Model file for the job. Use its own axes, mm. A direction names the side the tool comes from. Give positions to 0.01 mm unless a question says otherwise; leave off trailing zeros. Loops run counter-clockwise (first coordinate to the right, second up) from the corner with the lowest first, then second, coordinate; pieces in that order, holes last. Notation, with made-up numbers: (-12, 40) -> (35, 40) arc R23 ccw to (35, 60) -> close; hole circle Ø5 at (-21.75, 20.25). An arc over 180 degrees is marked (long way). Use CSV: the item, a comma, the result in double quotes. Start each with the question number.
(1) Pull direction X, two halves, no side cores. Call faces 5 (the flat face through (5, -37, -3)), 6 (the flat face through (0, -20, -22)), 7 (the flat face through (3, -37, 27.5)), 8 (the flat face through (-5, -37, -2)): pulls with the +X half, pulls with the -X half, needs draft (parallel to the pull), parting line crosses it, or undercut.
(2) 3-axis set-ups, long thin cutter, end or side, ignore diameter. For faces 1 (the cylindrical face through (-0.65, -65.14, -25.43)), 2 (the flat face through (0, -20, 23)), 3 (the cylindrical face through (-2.934, -35.548, -27.57)), 4 (the cylindrical face through (0.07, -48.974, -6.148)): which of +Z, -Z, +X, -X, +Y, -Y reach the whole face in a straight line?
(3) Flat gauge pins, fed straight in: pin 1 (2 mm diameter, centred on x = 2.5, y = -61, fed in from +Z); pin 2 (5.5 mm diameter, centred on x = 0, z = -22.5, fed in from +Y); pin 3 (3 mm diameter, centred on x = 1, z = -23, fed in from -Y). Where does each tip first touch, or does it go through?
(4) Cut at B-B on y = -18.5. Write the cut outline in (x, z).
(5) Drill centre lines: probe 1 along Y at (x, z) = (-2.5, -26.75); probe 2 along Z at (x, y) = (0.5, -15); probe 3 along Z at (x, y) = (2, -28). Where is each one in solid material? Low to high.
(6) Cut at A-A on z = -27.5. Write the cut outline in (x, y), then the cut area to 3 significant figures.
(7) Cut at D-D on y = -47.5. Write the cut outline in (x, z).
(8) Cut at C-C on z = -7.5. Write the cut outline in (x, y).
from build123d import *

# Parameters (mm, degrees)
F1_DEPTH  = 75
F3_R      = 2
F4_DEPTH  = 25
F6_R      = 3
F7_DEPTH  = 20
F8_R      = 3
F9_DEPTH  = 20
F10_R     = 3
F11_DEPTH = 20
F12_R     = 3
F13_DEPTH = 20
F2_R      = 2
F14_DEPTH = 10
F15_DEPTH = 25


with BuildPart() as f1:
    # F0 (on Front) → F1 (new body)
    with BuildSketch(Plane.XZ):
        Polygon((-5, 27.5), (-5, -32.5), (5, -32.5), (5, 27.5), (0, 27.5), (0, 32.5), align=None)
    extrude(amount=F1_DEPTH)

    # F3 (on face) → F4 (cut)
    with BuildSketch(Plane.YZ.offset(5)):
        with Locations((-47.5, -27.5)):
            Circle(F3_R)
        with Locations((-47.5, -7.5)):
            Circle(F3_R)
        with Locations((-27.5, -7.5)):
            Circle(F3_R)
        with Locations((-27.5, -27.5)):
            Circle(F3_R)
    extrude(amount=-F4_DEPTH, mode=Mode.SUBTRACT)

    # F6 (on face) → F7 (cut)
    with BuildSketch(Plane(origin=(0, 0, 0), x_dir=(-1, 0, 0), z_dir=(0, 1, 0))):
        with Locations((0, -22.5)):
            Circle(F6_R)
    extrude(amount=-F7_DEPTH, mode=Mode.SUBTRACT)

    # F8 (on face) → F9 (cut)
    with BuildSketch(Plane.XZ.offset(75)):
        with Locations((0, 22.5)):
            Circle(F8_R)
    extrude(amount=-F9_DEPTH, mode=Mode.SUBTRACT)

    # F10 (on face) → F11 (cut)
    with BuildSketch(Plane.XZ.offset(75)):
        with Locations((0, -22.5)):
            Circle(F10_R)
    extrude(amount=-F11_DEPTH, mode=Mode.SUBTRACT)

    # F12 (on face) → F13 (cut)
    with BuildSketch(Plane(origin=(0, 0, 0), x_dir=(-1, 0, 0), z_dir=(0, 1, 0))):
        with Locations((0, 22.5)):
            Circle(F12_R)
    extrude(amount=-F13_DEPTH, mode=Mode.SUBTRACT)

    # F2 (on face) → F14 (cut)
    with BuildSketch(Plane(origin=(0, 0, -32.5), x_dir=(1, 0, 0), z_dir=(0, 0, -1))):
        with Locations((-2.5, 37.5)):
            Circle(F2_R)
    extrude(amount=-F14_DEPTH, mode=Mode.SUBTRACT)

    # F3 (on face) → F15 (cut)
    with BuildSketch(Plane.YZ.offset(5)):
        with Locations((-47.5, -27.5)):
            Circle(F3_R)
        with Locations((-47.5, -7.5)):
            Circle(F3_R)
        with Locations((-27.5, -7.5)):
            Circle(F3_R)
        with Locations((-27.5, -27.5)):
            Circle(F3_R)
    extrude(amount=-F15_DEPTH, mode=Mode.SUBTRACT)


solid = f1.part
Check result:
1,face 5,"pulls with the +X half"
1,face 6,"undercut"
1,face 7,"needs draft"
1,face 8,"pulls with the -X half"
2,face 1,"-Y"
2,face 2,"+Y"
2,face 3,"-Z"
2,face 4,"+X, -X"
3,pin 1,"z = 27.5"
3,pin 2,"y = -20"
3,pin 3,"y = -55"
4,outline,"(-5, -32.5) -> (5, -32.5) -> (5, 27.5) -> (0, 27.5) -> (0, 32.5) -> (-5, 27.5) -> close; hole circle Ø6 at (0, -22.5); hole circle Ø6 at (0, 22.5)"
5,probe 1,"-75 to -49.35, -45.65 to -39.5, -35.5 to -29.35, -25.65 to 0"
5,probe 2,"-32.5 to -25.46, -19.54 to 19.54, 25.46 to 27.5"
5,probe 3,"-32.5 to -29.44, -25.56 to -9.44, -5.56 to 27.5"
6,outline,"(-5, -75) -> (5, -75) -> (5, -49.5) -> (-5, -49.5) -> close; (-5, -45.5) -> (5, -45.5) -> (5, -29.5) -> (-5, -29.5) -> close; (-5, -25.5) -> (5, -25.5) -> (5, 0) -> (-5, 0) -> close; hole circle Ø4 at (-2.5, -37.5)"
6,area,"657 mm²"
7,outline,"(-5, -32.5) -> (5, -32.5) -> (5, -29.5) -> (-5, -29.5) -> close; (-5, -25.5) -> (5, -25.5) -> (5, -9.5) -> (-5, -9.5) -> close; (-5, -5.5) -> (5, -5.5) -> (5, 27.5) -> (0, 27.5) -> (0, 32.5) -> (-5, 27.5) -> close"
8,outline,"(-5, -75) -> (5, -75) -> (5, -49.5) -> (-5, -49.5) -> close; (-5, -45.5) -> (5, -45.5) -> (5, -29.5) -> (-5, -29.5) -> close; (-5, -25.5) -> (5, -25.5) -> (5, 0) -> (-5, 0) -> close"
